from build123d import *

# Parameters (mm, degrees)
CYLINDER001_R     = 3.3725
CYLINDER001_DEPTH = 30
BOX008_W          = 23
BOX008_H          = 16
BOX008_DEPTH      = 6
BOX009_W          = 23
BOX009_H          = 57.5
BOX009_DEPTH      = 6
SKETCH_W          = 23
SKETCH_H          = 51.5
SKETCH_W_2        = 8
SKETCH_H_2        = 2
EXTRUDE_DEPTH     = 6


with BuildPart() as cylinder001:
    # Cylinder001 → Cylinder001 (new body)
    with BuildSketch(Plane.XZ.offset(-30)):
        Circle(CYLINDER001_R)
    extrude(amount=CYLINDER001_DEPTH)


with BuildPart() as cube008:
    # Box008 → Box008 (new body)
    with BuildSketch(Plane(origin=(-11.5, 7.25, -46), x_dir=(1, 0, 0), z_dir=(0, 0, 1))):
        with Locations((11.5, 8)):
            Rectangle(BOX008_W, BOX008_H)
    extrude(amount=BOX008_DEPTH)


with BuildPart() as cube009:
    # Box009 → Box009 (new body)
    with BuildSketch(Plane(origin=(-11.5, 17.25, 11.5), x_dir=(1, 0, 0), z_dir=(0, 1, 0))):
        with Locations((11.5, 28.75)):
            Rectangle(BOX009_W, BOX009_H)
    extrude(amount=BOX009_DEPTH)


with BuildPart() as mountplate:
    # Sketch → Extrude (new body)
    with BuildSketch(Plane(origin=(0, 0, 0), x_dir=(-1, 0, 0), z_dir=(0, 1, 0))):
        with Locations((0, -14.25)):
            Rectangle(SKETCH_W, SKETCH_H)
        with Locations((0, -12)):
            Rectangle(SKETCH_W_2, SKETCH_H_2, mode=Mode.SUBTRACT)
    extrude(amount=EXTRUDE_DEPTH)


with BuildPart() as mountplate_1:
    # Extrude placement: moved
    add(mountplate.part.moved(Location((0, 7.25, 0))))

    # Fusion003: union Cube008, Cube009
    add(cube008.part)
    add(cube009.part)

    # Cut002: cut Cylinder001
    add(cylinder001.part, mode=Mode.SUBTRACT)


solid = mountplate_1.part
Could you check a few things on this model? Use its own coordinates, in mm. A direction names the side the tool comes from. Give positions to 0.01 mm unless a question says otherwise; leave off trailing zeros. Order: outer loops, then holes, each group sorted by start corner. A loop starts at its lowest first (then second) coordinate and runs counter-clockwise, first axis right, second up. Notation, with made-up numbers: (44, 36.5) - (53, 36.5) arc R12 cw to (53, 57.5) - close; hole circle Ø7 at (74.25, 22). An arc over 180 degrees is marked (long way). One line per item, written item: value. Start each with the question number.
1. Imagine slicing it at A-A on z = -5.5. List the corners of the cut face in (x, y) for me, plus the area to 3 significant figures.
2. Thinking about a two-plate mould opening in Z: for faces 1 (the face through (-4, 10, -12)), 2 (the face through (0, 15, -46)), 3 (the face through (0, 7.25, -18)), which applies, +Z half, -Z half, draft (parallel to the pull), parting line (faces both ways), or undercut?
3. Imagine slicing it at D-D on y = 14.75. List the corners of the cut face in (x, z) for me, plus the area to 3 significant figures.
4. Imagine slicing it at C-C on x = -9. List the corners of the cut face in (y, z) for me.
5. If I drill on probe 1 along Z at (x, y) = (0, 9.15); probe 2 along X at (y, z) = (11.05, 0); probe 3 along Y at (x, z) = (4.75, 4), over which ranges is the centre line in solid material (lowest first)?
6. For faces 4 (the face through (0, 13.25, -14)), 5 (the face through (0, 23.25, -18)), 6 (the face through (4, 10, -12)), which set-ups out of +Z, -Z, +X, -X, +Y, -Y let a thin tool reach every point of the face, with its end or its side?
7. Imagine slicing it at B-B on x = 0. List the corners of the cut face in (y, z) for me.
Values:
1. outline: (-11.5, 7.25) - (11.5, 7.25) - (11.5, 13.25) - (-11.5, 13.25) - close; (-11.5, 17.25) - (11.5, 17.25) - (11.5, 23.25) - (-11.5, 23.25) - close
1. area: 276 mm²
2. face 1: undercut
2. face 2: -Z half
2. face 3: draft
3. outline: (-11.5, -46) - (11.5, -46) - (11.5, -40) - (-11.5, -40) - close
3. area: 138 mm²
4. outline: (7.25, -46) - (23.25, -46) - (23.25, 11.5) - (17.25, 11.5) - (17.25, -40) - (13.25, -40) - (13.25, 11.5) - (7.25, 11.5) - close
5. probe 1: -46 to -13, -11 to -3.37, 3.37 to 11.5
5. probe 2: -11.5 to -3.37, 3.37 to 11.5
5. probe 3: 7.25 to 13.25, 17.25 to 23.25
6. face 4: +Z, +X, -X
6. face 5: +Z, -Z, +X, -X, +Y
6. face 6: -Y
7. outline: (7.25, -46) - (23.25, -46) - (23.25, -3.37) - (17.25, -3.37) - (17.25, -40) - (13.25, -40) - (13.25, -13) - (7.25, -13) - close; (7.25, -11) - (13.25, -11) - (13.25, -3.37) - (7.25, -3.37) - close; (7.25, 3.37) - (13.25, 3.37) - (13.25, 11.5) - (7.25, 11.5) - close; (17.25, 3.37) - (23.25, 3.37) - (23.25, 11.5) - (17.25, 11.5) - close
